Verification items for the finished model (mm, model axes). Face numbers are marked on the shaded views. A direction names the side the tool comes from. Give positions to 0.01 mm unless a question says otherwise; leave off trailing zeros. Order: outer loops, then holes, each group sorted by start corner. A loop starts at its lowest first (then second) coordinate and runs counter-clockwise, first axis right, second up.
(1) Scan lines: L1, parallel to Z at x = 79.55, y = 27; L2, parallel to Y at x = 25, z = 14.25; L3, parallel to X at y = 19.5, z = 3.5. Record each from-to range of solid material in increasing order.
(2) Access from +Z, -Z, +X, -X, +Y, -Y to the whole of each face (thin tool, end or side, straight path). Record for the marked faces 4 and 5.
(3) Sectioned sample at B-B on y = 15.5. Record the cut outline in (x, z), plus the area to 3 significant figures.
(4) Mould release check, pull along X, two halves, no side actions. Record for the marked faces 1, 2 and 3: pulls with the +X half, pulls with the -X half, needs draft (parallel to the pull), parting line crosses it, or undercut.
(5) Sectioned sample at D-D on z = 15.5. Record the cut outline in (x, y).
(6) Sectioned sample at C-C on x = 17.5. Record the cut outline in (y, z).
(7) Sectioned sample at A-A on x = 44. Record the cut outline in (y, z), plus the area to 3 significant figures.
```python
from build123d import *

# Parameters (mm, degrees)
CYLINDER033_R     = 8
CYLINDER033_DEPTH = 10
CYLINDER034_R     = 8
CYLINDER034_DEPTH = 10
CYLINDER042_R     = 8
CYLINDER042_DEPTH = 10
PAD_DEPTH         = 24


with BuildPart() as b_w:
    # Cylinder033 → Cylinder033 (new body)
    with BuildSketch(Plane(origin=(5, 15.5, 15.5), x_dir=(0, 0, 1), z_dir=(-1, 0, 0))):
        Circle(CYLINDER033_R)
    extrude(amount=CYLINDER033_DEPTH)


with BuildPart() as b_o:
    # Cylinder034 → Cylinder034 (new body)
    with BuildSketch(Plane(origin=(85, 27, 15.5), x_dir=(0, 0, 1), z_dir=(-1, 0, 0))):
        Circle(CYLINDER034_R)
    extrude(amount=CYLINDER034_DEPTH)


with BuildPart() as b_n001:
    # Cylinder042 → Cylinder042 (new body)
    with BuildSketch(Plane(origin=(44, 38, 15.5), x_dir=(0, 0, 1), z_dir=(0, 1, 0))):
        Circle(CYLINDER042_R)
    extrude(amount=CYLINDER042_DEPTH)


with BuildPart() as cut034:
    # Sketch → Pad (new body)
    with BuildSketch(Plane.XY):
        with BuildLine():
            Line((11, 0), (69, 0))
            ThreePointArc((69, 0), (76.778175, 3.221825), (80, 11))
            Line((80, 11), (80, 32))
            ThreePointArc((80, 32), (76.778175, 39.778175), (69, 43))
            Line((69, 43), (11, 43))
            ThreePointArc((11, 43), (3.221825, 39.778175), (0, 32))
            Line((0, 32), (0, 11))
            ThreePointArc((0, 11), (3.221825, 3.221825), (11, 0))
        make_face()
        with BuildLine():
            Line((11, 1), (69, 1))
            ThreePointArc((69, 1), (76.071068, 3.928932), (79, 11))
            Line((79, 11), (79, 32))
            ThreePointArc((79, 32), (76.071068, 39.071068), (69, 42))
            Line((69, 42), (11, 42))
            ThreePointArc((11, 42), (3.928932, 39.071068), (1, 32))
            Line((1, 32), (1, 11))
            ThreePointArc((1, 11), (3.928932, 3.928932), (11, 1))
        make_face(mode=Mode.SUBTRACT)
    extrude(amount=PAD_DEPTH)

    # Cut032: cut B_N001
    add(b_n001.part, mode=Mode.SUBTRACT)

    # Cut033: cut B_O
    add(b_o.part, mode=Mode.SUBTRACT)

    # Cut034: cut B_W
    add(b_w.part, mode=Mode.SUBTRACT)


solid = cut034.part
```
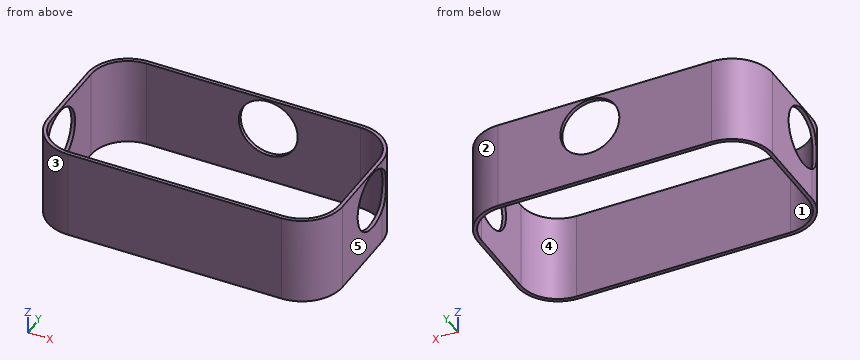
Ans:
1. L1: z = 0 to 7.5, 23.5 to 24
1. L2: y = 0 to 1, 42 to 43
1. L3: x = 0 to 1, 79 to 80
2. face 4: +Z, -Z
2. face 5: +Z, -Z, +X, +Y, -Y
3. outline: (0, 0) - (1, 0) - (1, 7.5) - (0, 7.5) - close; (0, 23.5) - (1, 23.5) - (1, 24) - (0, 24) - close; (79, 0) - (80, 0) - (80, 24) - (79, 24) - close
3. area: 32.0 mm2
4. face 1: undercut
4. face 2: pulls with the +X half
4. face 3: pulls with the -X half
5. outline: (0, 23.5) - (1, 23.5) - (1, 32) arc R10 cw to (11, 42) - (36, 42) - (36, 43) - (11, 43) arc R11 ccw to (0, 32) - close; (0.57, 7.5) arc R11 ccw to (11, 0) - (69, 0) arc R11 ccw to (80, 11) - (80, 19) - (79, 19) - (79, 11) arc R10 cw to (69, 1) - (11, 1) arc R10 cw to (1.63, 7.5) - close; (52, 42) - (69, 42) arc R10 cw to (78.54, 35) - (79.58, 35) arc R11 ccw to (69, 43) - (52, 43) - close
6. outline: (0, 0) - (1, 0) - (1, 24) - (0, 24) - close; (42, 0) - (43, 0) - (43, 24) - (42, 24) - close
7. outline: (0, 0) - (1, 0) - (1, 24) - (0, 24) - close; (42, 0) - (43, 0) - (43, 7.5) - (42, 7.5) - close; (42, 23.5) - (43, 23.5) - (43, 24) - (42, 24) - close
7. area: 32.0 mm2
